The listing builds one solid part. Answer for the finished solid, in the listing's coordinates (mm). A direction names the side the tool comes from. Coordinates: 2 decimals unless noted, no trailing zeros. Loops run counter-clockwise (first coordinate to the right, second up) from the corner with the lowest first, then second, coordinate; pieces in that order, holes last. Notation, with made-up numbers: M 34,41 L 60,41 A12 ccw 60,46 Z; hole C 6.5,16 d2. An arc over 180 degrees is marked long. Answer as a JSON object with one key per item and string values. Group by question number.
1. For faces 1 (the face through (1934.218, 998, 1)), 2 (the face through (1916, 1015.065, 1)), 3 (the face through (1963, 1005.065, 1)), determine the directions among +Z, -Z, +X, -X, +Y, -Y from which every point of the face is accessible in a straight line to the end or side of a thin tool.
2. Determine the mould class of faces 4 (the face through (1956.718, 998, 1)), 5 (the face through (1919, 973.907, 1)), 6 (the face through (1932.06, 973, 1)) for opening direction Y: released by +Y, released by -Y, zero draft, split by the parting line, or undercut.
3. A cutting plane is placed at B-B on x = 1952. Give the vertices of the cut face in (y, z), and give its area (3 significant figures).
4. A cutting plane is placed at C-C on y = 993. Give the vertices of the cut face in (x, z), and give its area (3 significant figures).
5. A cutting plane is placed at D-D on z = 1.1. State how many separate pieces and enclosed holes the cut face has, and give its area (3 significant figures).
6. Given pin 1 (0.8 mm diameter, centred on x = 1960, z = 0.5, fed in from -Y); pin 2 (0.8 mm diameter, centred on y = 978, z = 0.5, fed in from -X); pin 3 (0.8 mm diameter, centred on x = 1959.5, z = 0.5, fed in from +Y), each flat-ended and moving along its own axis, determine where each tip first touches the part or whether it passes through.
7. A cutting plane is placed at A-A on y = 1006. Give the vertices of the cut face in (x, z).
8. Straight lines are drawn through the part: L1, parallel to X at y = 1002, z = 0.7; L2, parallel to Y at x = 1948, z = 0.95; L3, parallel to X at y = 985.5, z = 1.1. For each, find the intervals that lie inside material, in ascending order.
from build123d import *

# Parameters (mm, degrees)
EXTRUDE_1_DEPTH = 1.5


with BuildPart() as part:
    # 草图1 → 凸台-拉伸1 (new body)
    with BuildSketch(Plane.XY):
        Polygon((1932.059632511, 1023.906869704), (1922.059632511, 1023.906869704), (1922.059632511, 1021.906869704), (1916.717816775, 1021.906869704), (1916.717816775, 1015.065053968), (1914.717816775, 1015.065053968), (1914.717816775, 1005.065053968), (1916.717816775, 1005.065053968), (1916.717816775, 990.748685439), (1914.717816775, 990.748685439), (1914.717816775, 980.748685439), (1916.717816775, 980.748685439), (1916.717816775, 973.906869704), (1922.059632511, 973.906869704), (1922.059632511, 971.906869704), (1932.059632511, 971.906869704), (1932.059632511, 973.906869704), (1946.376001039, 973.906869704), (1946.376001039, 971.906869704), (1956.376001039, 971.906869704), (1956.376001039, 973.906869704), (1961.717816775, 973.906869704), (1961.717816775, 980.748685439), (1963.717816775, 980.748685439), (1963.717816775, 990.748685439), (1961.717816775, 990.748685439), (1961.717816775, 1005.065053968), (1963.717816775, 1005.065053968), (1963.717816775, 1015.065053968), (1961.717816775, 1015.065053968), (1961.717816775, 1021.906869704), (1956.376001039, 1021.906869704), (1956.376001039, 1023.906869704), (1946.376001039, 1023.906869704), (1946.376001039, 1021.906869704), (1932.059632511, 1021.906869704), align=None)
        with BuildLine():
            Line((1921.717816775, 1013.906869704), (1921.717816775, 981.906869704))
            ThreePointArc((1921.717816775, 981.906869704), (1922.596496432, 979.78554936), (1924.717816775, 978.906869704))
            Line((1924.717816775, 978.906869704), (1931.217816775, 978.906869704))
            ThreePointArc((1931.217816775, 978.906869704), (1933.339137119, 979.78554936), (1934.217816775, 981.906869704))
            Line((1934.217816775, 981.906869704), (1934.217816775, 1013.906869704))
            ThreePointArc((1934.217816775, 1013.906869704), (1933.339137119, 1016.028190047), (1931.217816775, 1016.906869704))
            Line((1931.217816775, 1016.906869704), (1924.717816775, 1016.906869704))
            ThreePointArc((1924.717816775, 1016.906869704), (1922.596496432, 1016.028190047), (1921.717816775, 1013.906869704))
        make_face(mode=Mode.SUBTRACT)
        with BuildLine():
            Line((1956.717816775, 1013.906869704), (1956.717816775, 981.906869704))
            ThreePointArc((1956.717816775, 981.906869704), (1955.839137119, 979.78554936), (1953.717816775, 978.906869704))
            Line((1953.717816775, 978.906869704), (1947.217816775, 978.906869704))
            ThreePointArc((1947.217816775, 978.906869704), (1945.096496432, 979.78554936), (1944.217816775, 981.906869704))
            Line((1944.217816775, 981.906869704), (1944.217816775, 1013.906869704))
            ThreePointArc((1944.217816775, 1013.906869704), (1945.096496432, 1016.028190047), (1947.217816775, 1016.906869704))
            Line((1947.217816775, 1016.906869704), (1953.717816775, 1016.906869704))
            ThreePointArc((1953.717816775, 1016.906869704), (1955.839137119, 1016.028190047), (1956.717816775, 1013.906869704))
        make_face(mode=Mode.SUBTRACT)
    extrude(amount=EXTRUDE_1_DEPTH)


solid = part.part
From the geometry:
{
 "1": {"face 1": "+Z, -Z", "face 2": "+Z, -Z, -X, +Y", "face 3": "+Z, -Z, +X"},
 "2": {"face 4": "undercut", "face 5": "released by -Y", "face 6": "zero draft"},
 "3": {"outline": "M 971.91,0 L 978.91,0 L 978.91,1.5 L 971.91,1.5 Z; M 1016.91,0 L 1023.91,0 L 1023.91,1.5 L 1016.91,1.5 Z", "area": "21.0 mm²"},
 "4": {"outline": "M 1916.72,0 L 1921.72,0 L 1921.72,1.5 L 1916.72,1.5 Z; M 1934.22,0 L 1944.22,0 L 1944.22,1.5 L 1934.22,1.5 Z; M 1956.72,0 L 1961.72,0 L 1961.72,1.5 L 1956.72,1.5 Z", "area": "30.0 mm²"},
 "5": {"separate pieces": "1", "enclosed holes": "2", "area": "1,390 mm²"},
 "6": {"pin 1": "stops at y = 973.91", "pin 2": "stops at x = 1916.72", "pin 3": "stops at y = 1021.91"},
 "7": {"outline": "M 1914.72,0 L 1921.72,0 L 1921.72,1.5 L 1914.72,1.5 Z; M 1934.22,0 L 1944.22,0 L 1944.22,1.5 L 1934.22,1.5 Z; M 1956.72,0 L 1963.72,0 L 1963.72,1.5 L 1956.72,1.5 Z"},
 "8": {"L1": "x = 1916.72 to 1921.72, 1934.22 to 1944.22, 1956.72 to 1961.72", "L2": "y = 971.91 to 978.91, 1016.91 to 1023.91", "L3": "x = 1914.72 to 1921.72, 1934.22 to 1944.22, 1956.72 to 1963.72"}
}
